CAD build for the part. Positions are in the model's coordinates, mm. Face numbers are marked on the shaded views. A direction names the side the tool comes from. Coordinates: 2 decimals unless noted, no trailing zeros. Order: outer loops, then holes, each group sorted by start corner. A loop starts at its lowest first (then second) coordinate and runs counter-clockwise, first axis right, second up. Notation, with made-up numbers: M 53.25,-24 L 78.25,-24 A16 cw 78.25,3 Z; hole C 61,5.5 d10. An arc over 180 degrees is marked long. One line per item, written item: value.
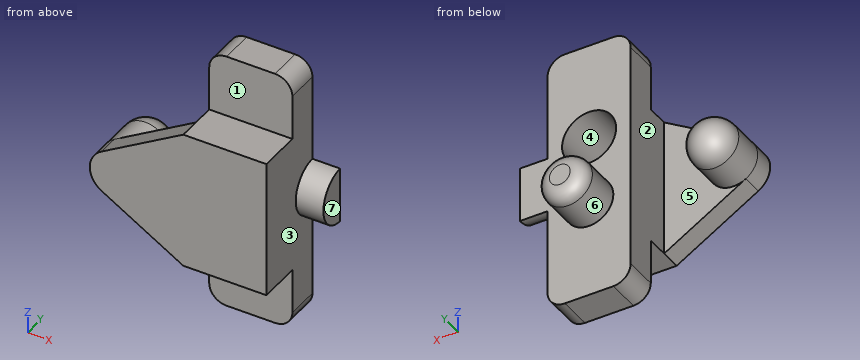
from build123d import *

# Parameters (mm, degrees)
BOSS_EXTRUDE1_DEPTH = 1.5
BOSS_EXTRUDE2_START = 4
SKETCH2_R           = 1.75
SKETCH2_W           = 6
SKETCH2_H           = 10
BOSS_EXTRUDE2_DEPTH = 4
BOSS_EXTRUDE3_DEPTH = 2.4
FILLET1_R           = 1.75
SKETCH4_R           = 1.75
BOSS_EXTRUDE4_DEPTH = 3.5
FILLET2_R           = 1
SKETCH5_R           = 1.95
CUT_EXTRUDE1_DEPTH  = 3.75
BOSS_EXTRUDE5_DEPTH = 2


with BuildPart() as part:
    # Sketch1 → Boss-Extrude1 (new body)
    with BuildSketch(Plane(origin=(0, 0, 0), x_dir=(1, 0, 0), z_dir=(0, 1, 0))):
        with BuildLine():
            Line((5, 5), (11, 5))
            Line((11, 5), (11, -5))
            Line((11, -5), (5, -5))
            Line((5, -5), (-0.892691591, -1.505191591))
            ThreePointArc((-0.892691591, -1.505191591), (-1.75, 0), (-0.892691591, 1.505191591))
            Line((-0.892691591, 1.505191591), (5, 5))
        make_face()
    extrude(amount=-BOSS_EXTRUDE1_DEPTH)

    # Sketch2 → Boss-Extrude2 (add)
    with BuildSketch(Plane(origin=(0, 0, 0), x_dir=(1, 0, 0), z_dir=(0, 1, 0)).offset(BOSS_EXTRUDE2_START)):
        with Locations(Location((0, 0, 0), (0, 0, 270))):
            Circle(SKETCH2_R)
        with Locations((8, 0)):
            Rectangle(SKETCH2_W, SKETCH2_H)
    extrude(amount=-BOSS_EXTRUDE2_DEPTH)

    # Sketch3 → Boss-Extrude3 (add)
    with BuildSketch(Plane(origin=(0, 4, 0), x_dir=(1, 0, 0), z_dir=(0, 1, 0))):
        with BuildLine():
            Line((5, 5), (11, 5))
            Line((11, 5), (11, 8.25))
            ThreePointArc((11, 8.25), (10.633883476, 9.133883476), (9.75, 9.5))
            Line((9.75, 9.5), (6.25, 9.5))
            ThreePointArc((6.25, 9.5), (5.366116524, 9.133883476), (5, 8.25))
            Line((5, 8.25), (5, 5))
        make_face()
        with BuildLine():
            Line((5, -5), (11, -5))
            Line((11, -5), (11, -8.25))
            ThreePointArc((11, -8.25), (10.633883476, -9.133883476), (9.75, -9.5))
            Line((9.75, -9.5), (6.25, -9.5))
            ThreePointArc((6.25, -9.5), (5.366116524, -9.133883476), (5, -8.25))
            Line((5, -8.25), (5, -5))
        make_face()
    extrude(amount=-BOSS_EXTRUDE3_DEPTH)

    # Fillet1
    fillet1_edges = [part.edges().sort_by_distance(p)[0] for p in [
        (0, 4, -1.75),
    ]]
    fillet(fillet1_edges, radius=FILLET1_R)

    # Sketch4 → Boss-Extrude4 (add)
    with BuildSketch(Plane(origin=(0, 4, 0), x_dir=(1, 0, 0), z_dir=(0, 1, 0))):
        with Locations(Location((8, 2.5, 0), (0, 0, 270))):
            Circle(SKETCH4_R)
    extrude(amount=BOSS_EXTRUDE4_DEPTH)

    # Fillet2
    fillet2_edges = [part.edges().sort_by_distance(p)[0] for p in [
        (8, 7.5, -4.25),
    ]]
    fillet(fillet2_edges, radius=FILLET2_R)

    # Sketch5 → Cut-Extrude1 (cut)
    with BuildSketch(Plane(origin=(0, 4, 0), x_dir=(1, 0, 0), z_dir=(0, 1, 0))):
        with Locations(Location((8, -2.5, 0), (0, 0, 270))):
            Circle(SKETCH5_R)
    extrude(amount=-CUT_EXTRUDE1_DEPTH, mode=Mode.SUBTRACT)

    # Sketch6 → Boss-Extrude5 (add)
    with BuildSketch(Plane(origin=(11, 0, 0), x_dir=(0, 0, -1), z_dir=(1, 0, 0))):
        with BuildLine():
            Line((-2, 4), (2, 4))
            ThreePointArc((2, 4), (0, 2), (-2, 4))
        make_face()
    extrude(amount=BOSS_EXTRUDE5_DEPTH)


solid = part.part
Q1. Mould opens along X. For the marked faces 4, 5, 6 and 7 say: released by +X, released by -X, zero draft, split by the parting line, or undercut.
Recorded:
face 4: undercut
face 5: undercut
face 6: split by the parting line
face 7: released by +X
Q2. Which spindle directions (+Z, -Z, +X, -X, +Y, -Y) get a long thin tool onto all of the face, cutting with end or side? Do the marked faces 1, 2 and 3. Say none if no direction does.
Recorded:
face 1: +Z, +X, -X, -Y
face 2: +Z, -Z, +Y
face 3: +X, -Y
Q3. Slice it at B-B (z = 0). List the corners of the cut face in (x, y), plus the area to 3 significant figures.
Recorded:
outline: M -1.75,-1.5 L 11,-1.5 L 11,2 L 13,2 L 13,4 L 5,4 L 5,0 L 1.75,0 L 1.75,2.25 A1.75 ccw -1.75,2.25 Z
area: 59.8 mm^2
Q4. Drill centre lines: line 1 along X through (y, z) = (1.8, 2.5); line 2 along Y through (x, z) = (4.5, -1); line 3 along X through (y, z) = (3, 4). Where is each one in solid material? Low to high.
Recorded:
line 1: x = 5 to 6.05, 9.95 to 11
line 2: y = -1.5 to 0
line 3: x = 5 to 6.75, 9.25 to 11
Q5. Slice it at A-A (y = 1). List the corners of the cut face in (x, z), plus the area to 3 significant figures.
Recorded:
outline: C 0,0 d3.5; M 5,-5 L 11,-5 L 11,5 L 5,5 Z; hole C 8,2.5 d3.9
area: 57.7 mm^2
Q6. Pin check, flat tips, straight feed: pin 1 Ø3 at (x, z) = (6.5, 5.5) entering from +Y; pin 2 Ø1.6 at (x, y) = (7, 0) entering from -Z; pin 3 Ø5 at (x, z) = (11, -4.5) entering from +Y; pin 4 Ø1 at (y, z) = (6, 4) entering from +X. Stop position of each tip, or through.
Recorded:
pin 1: stops at y = 4
pin 2: stops at z = -5
pin 3: stops at y = 7.43
pin 4: passes through
Q7. Slice it at D-D (y = 4.25). List the corners of the cut face in (x, z).
Recorded:
outline: C 8,-2.5 d3.5
Q8. Slice it at C-C (x = 1). List the corners of the cut face in (y, z), plus the area to 3 significant figures.
Recorded:
outline: M -1.5,-2.63 L 0,-2.63 L 0,-1.44 L 2.25,-1.44 A1.44 ccw 2.25,1.44 L 0,1.44 L 0,2.63 L -1.5,2.63 Z
area: 17.6 mm^2
